```python
from build123d import *

# Parameters (mm, degrees)
BOX019_W     = 22
BOX019_H     = 27
BOX019_DEPTH = 10
BOX016_W     = 43.3
BOX016_H     = 27
BOX016_DEPTH = 43.3
BOX015_W     = 48.3
BOX015_H     = 30
BOX015_DEPTH = 48.3


with BuildPart() as cube:
    # Box019 → Box019 (new body)
    with BuildSketch(Plane(origin=(47.85, 68.5, -75), x_dir=(1, 0, 0), z_dir=(0, 0, 1))):
        with Locations((11, 13.5)):
            Rectangle(BOX019_W, BOX019_H)
    extrude(amount=BOX019_DEPTH)


with BuildPart() as statictraynegative:
    # Box016 → Box016 (new body)
    with BuildSketch(Plane(origin=(93.5, 0, 2.5), x_dir=(1, 0, 0), z_dir=(0, 0, 1))):
        with Locations((21.65, 13.5)):
            Rectangle(BOX016_W, BOX016_H)
    extrude(amount=BOX016_DEPTH)


with BuildPart() as lineartray:
    # Box015 → Box015 (new body)
    with BuildSketch(Plane(origin=(91, 0, 0), x_dir=(1, 0, 0), z_dir=(0, 0, 1))):
        with Locations((24.15, 15)):
            Rectangle(BOX015_W, BOX015_H)
    extrude(amount=BOX015_DEPTH)

    # Cut017: cut StaticTrayNegative
    add(statictraynegative.part, mode=Mode.SUBTRACT)


with BuildPart() as lineartray_1:
    # Cut017 placement: moved
    add(lineartray.part.moved(Location((-56.3, 68.5, -71))))

    # Cut018: cut Cube
    add(cube.part, mode=Mode.SUBTRACT)


solid = lineartray_1.part
```
Could you check a few things on this model? Use its own coordinates, in mm. A direction names the side the tool comes from. Round coordinates to 2 decimals unless told otherwise and drop trailing zeros. Write each loop counter-clockwise with the first axis right and the second up, starting at its lowest first coordinate (ties: lowest second). Pieces come first, ordered by that corner, then holes.
(1) Thinking about a two-plate mould opening in Z: for faces 1 (the face through (59, 98.5, -47)), 2 (the face through (37.2, 82, -47)), 3 (the face through (59, 97, -71)), which applies, +Z half, -Z half, draft (parallel to the pull), parting line (faces both ways), or undercut?
Findings below:
face 1: draft
face 2: undercut
face 3: -Z half
(2) Which directions (+Z, -Z, +X, -X, +Y, -Y) give clear straight access to the entire face, cutting with the end or side of a thin tool? Please do faces 4 (the face through (83, 83, -47)), 5 (the face through (59, 82, -25.2)), 6 (the face through (69.85, 82, -70)).
Findings below:
face 4: +Z, -Z, +X, +Y, -Y
face 5: -Y
face 6: -Z, -Y
(3) Suppose I cut it at D-D on x = 65.5. Write out the boundary of the cut face in (y, z), and give its area (3 significant figures).
Findings below:
outline: (68.5, -25.2) - (95.5, -25.2) - (95.5, -71) - (98.5, -71) - (98.5, -22.7) - (68.5, -22.7) - close
area: 212 mm2
(4) For pin 1 (13 mm diameter, centred on x = 65, z = -39.5, fed in from -Y); pin 2 (8 mm diameter, centred on x = 43.5, z = -65, fed in from -Y), each with a flat end and sliding along its axis, tell me the tip position at first contact or that it passes through.
Findings below:
pin 1: stops at y = 95.5
pin 2: stops at y = 68.5
(5) Suppose I cut it at C-C on z = -41. Write out the boundary of the cut face in (x, y), and give its area (3 significant figures).
Findings below:
outline: (34.7, 68.5) - (37.2, 68.5) - (37.2, 95.5) - (80.5, 95.5) - (80.5, 68.5) - (83, 68.5) - (83, 98.5) - (34.7, 98.5) - close
area: 280 mm2
(6) If I drill on probe 1 along X at (y, z) = (86, -52.5); probe 2 along Z at (x, y) = (72, 78.75); probe 3 along Y at (x, z) = (73, -47), over which ranges is the centre line in solid material (lowest first)?
Findings below:
probe 1: x = 34.7 to 37.2, 80.5 to 83
probe 2: z = -71 to -68.5, -25.2 to -22.7
probe 3: y = 95.5 to 98.5
(7) Suppose I cut it at B-B on x = 42.5. Write out the boundary of the cut face in (y, z).
Findings below:
outline: (68.5, -71) - (98.5, -71) - (98.5, -22.7) - (68.5, -22.7) - (68.5, -25.2) - (95.5, -25.2) - (95.5, -68.5) - (68.5, -68.5) - close
(8) Suppose I cut it at A-A on y = 72.75. Write out the boundary of the cut face in (x, z).
Findings below:
outline: (34.7, -71) - (47.85, -71) - (47.85, -68.5) - (37.2, -68.5) - (37.2, -25.2) - (80.5, -25.2) - (80.5, -68.5) - (69.85, -68.5) - (69.85, -71) - (83, -71) - (83, -22.7) - (34.7, -22.7) - close
